CAD build for the part. Positions are in the model's coordinates, mm. Coordinates: 2 decimals unless noted, no trailing zeros. Write each loop counter-clockwise with the first axis right and the second up, starting at its lowest first coordinate (ties: lowest second). Pieces come first, ordered by that corner, then holes. Notation, with made-up numbers: M -21,53 L 16,53 A32 ccw 16,79 Z; hole C 18,78.25 d11. An arc over 180 degrees is marked long. Put each result on its own line as item: value. Start each with the question number.
```python
from build123d import *

# Parameters (mm, degrees)
SKETCH1_RX          = 30
SKETCH1_RY          = 20
BOSS_EXTRUDE1_DEPTH = 30
FILLET1_R           = 10


with BuildPart() as part:
    # Sketch1 → Boss-Extrude1 (new body)
    with BuildSketch(Plane(origin=(0, 0, 0), x_dir=(1, 0, 0), z_dir=(0, 1, 0))):
        Polygon((25, 40), (-25, 40), (-40, 0), (-17.5, -30), (17.5, -30), (40, 0), align=None)
        with Locations(Location((0, 0), (0, 0, -180))):
            Ellipse(SKETCH1_RX, SKETCH1_RY, mode=Mode.SUBTRACT)
    extrude(amount=BOSS_EXTRUDE1_DEPTH)

    # Fillet1
    fillet1_edges = [part.edges().sort_by_distance(p)[0] for p in [
        (-25, 15, -40),
        (25, 15, -40),
        (40, 15, 0),
        (17.5, 15, 30),
        (-17.5, 15, 30),
        (-40, 15, 0),
    ]]
    fillet(fillet1_edges, radius=FILLET1_R)


solid = part.part
```
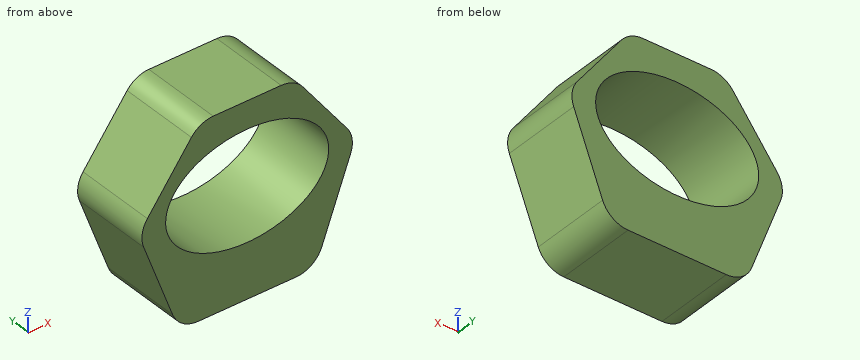
(1) Drop flat-ended pins along their axis: pin 1 (4 mm diameter, centred on x = -28, y = 7.5, fed in from +Z); pin 2 (10 mm diameter, centred on y = 11.5, z = -30.5, fed in from -X); pin 3 (1 mm diameter, centred on y = 23, z = -2.5, fed in from -X). Give the stop position or say it passes through.
(2) Drill centre lines: line 1 (Z direction, x = 6, y = 13.75); line 2 (X direction, y = 8.25, z = -10.5); line 3 (Z direction, x = -6.5, y = 20). Where is each one in solid material? Low to high. Write a range as [from, to].
(3) Slice it at B-B, the plane x = 33.5. Write the cut outline in (y, z).
(4) Slice it at A-A, the plane z = -22. Write the cut outline in (x, y), then the cut area to 4 significant figures.
Result set:
1. pin 1: stops at z = 18.67
1. pin 2: stops at x = -30.44
1. pin 3: stops at x = -38.71
2. line 1: z = [-40, -19.6], [19.6, 30]
2. line 2: x = [-36.06, -25.53], [25.53, 36.06]
2. line 3: z = [-40, -19.52], [19.52, 30]
3. outline: M 0,-17.33 L 30,-17.33 L 30,8.67 L 0,8.67 Z
4. outline: M -31.75,0 L 31.75,0 L 31.75,30 L -31.75,30 Z
4. area: 1,905 mm^2
